from build123d import *

# Parameters (mm, degrees)
ESQUISSE1_R                                  = 5
BOSS_EXTRU_1_DEPTH                           = 5
CHAMBRAGE_POUR_VIS_T_TE_RONDE_BOMB_E_A_COUNT = 2
CHAMBRAGE_POUR_VIS_T_TE_RONDE_BOMB_E_A_PITCH = 152
CHAMBRAGE_POUR_VIS_T_TE_RONDE_BOMB_2_COUNT   = 2
CHAMBRAGE_POUR_VIS_T_TE_RONDE_BOMB_2_PITCH   = 111
CHAMBRAGE_POUR_VIS_T_TE_RONDE_BOMB_3_COUNT   = 2
CHAMBRAGE_POUR_VIS_T_TE_RONDE_BOMB_3_PITCH   = 188.215302247
CHAMBRAGE_POUR_VIS_T_TE_RONDE_BOMB_4_A_COUNT = 2
CHAMBRAGE_POUR_VIS_T_TE_RONDE_BOMB_4_A_PITCH = 152
CHAMBRAGE_POUR_VIS_T_TE_RONDE_BOMB_5_COUNT   = 2
CHAMBRAGE_POUR_VIS_T_TE_RONDE_BOMB_5_PITCH   = 111
CHAMBRAGE_POUR_VIS_T_TE_RONDE_BOMB_6_COUNT   = 2
CHAMBRAGE_POUR_VIS_T_TE_RONDE_BOMB_6_PITCH   = 188.215302247


with BuildPart() as part:
    # Esquisse1 → Boss.-Extru.1 (new body)
    with BuildSketch(Plane(origin=(0, 0, 0), x_dir=(1, 0, 0), z_dir=(0, 1, 0))):
        with Locations(Location((0, 0, 0), (0, 0, 270))):
            Circle(ESQUISSE1_R)
    extrude(amount=BOSS_EXTRU_1_DEPTH)

    # Esquisse3 → Chambrage pour vis _ t_te ronde bomb_e (revolve, cut)
    with BuildSketch(Plane(origin=(0, 11, -152), x_dir=(0, 0, 1), z_dir=(1, 0, 0))):
        Polygon((0, 0), (0, 6.839402285), (1.397, 6), (1.397, 1.8034), (2.77876, 1.8034), (2.77876, 0.635), (3.41376, 0), align=None)
    chambrage_pour_vis_t_te_ronde_bomb_e = revolve(axis=Axis((0, 17.35, -152), (0, -1, 0)), mode=Mode.SUBTRACT)

    # Chambrage pour vis _ t_te ronde bomb_e a: Chambrage pour vis _ t_te ronde bomb_e ×2
    with Locations(*[(0, 0, i * CHAMBRAGE_POUR_VIS_T_TE_RONDE_BOMB_E_A_PITCH) for i in range(1, CHAMBRAGE_POUR_VIS_T_TE_RONDE_BOMB_E_A_COUNT)]):
        add(chambrage_pour_vis_t_te_ronde_bomb_e, mode=Mode.SUBTRACT)

    # Chambrage pour vis _ t_te ronde bomb 2: Chambrage pour vis _ t_te ronde bomb_e ×2
    with Locations(*[(i * CHAMBRAGE_POUR_VIS_T_TE_RONDE_BOMB_2_PITCH, 0, 0) for i in range(1, CHAMBRAGE_POUR_VIS_T_TE_RONDE_BOMB_2_COUNT)]):
        add(chambrage_pour_vis_t_te_ronde_bomb_e, mode=Mode.SUBTRACT)

    # Chambrage pour vis _ t_te ronde bomb 3: Chambrage pour vis _ t_te ronde bomb_e ×2
    with Locations(*[Vector(0.5897501354816591, 0, 0.8075857711100195) * (i * CHAMBRAGE_POUR_VIS_T_TE_RONDE_BOMB_3_PITCH) for i in range(1, CHAMBRAGE_POUR_VIS_T_TE_RONDE_BOMB_3_COUNT)]):
        add(chambrage_pour_vis_t_te_ronde_bomb_e, mode=Mode.SUBTRACT)

    # Esquisse5 → Chambrage pour vis _ t_te ronde bomb 4 (revolve, cut)
    with BuildSketch(Plane(origin=(0, 11, 0), x_dir=(0, 0, 1), z_dir=(1, 0, 0))):
        Polygon((0, 0), (0, 6.839402285), (1.397, 6), (1.397, 1.8034), (2.77876, 1.8034), (2.77876, 0.635), (3.41376, 0), align=None)
    chambrage_pour_vis_t_te_ronde_bomb_4 = revolve(axis=Axis((0, 17.35, 0), (0, -1, 0)), mode=Mode.SUBTRACT)

    # Chambrage pour vis _ t_te ronde bomb 4 a: Chambrage pour vis _ t_te ronde bomb 4 ×2
    with Locations(*[Vector(-0.4987370820513642, 0, -0.8667533230319286) * (i * CHAMBRAGE_POUR_VIS_T_TE_RONDE_BOMB_4_A_PITCH) for i in range(1, CHAMBRAGE_POUR_VIS_T_TE_RONDE_BOMB_4_A_COUNT)]):
        add(chambrage_pour_vis_t_te_ronde_bomb_4, mode=Mode.SUBTRACT)

    # Chambrage pour vis _ t_te ronde bomb 5: Chambrage pour vis _ t_te ronde bomb 4 ×2
    with Locations(*[Vector(-0.8667533230319285, 0, 0.4987370820513645) * (i * CHAMBRAGE_POUR_VIS_T_TE_RONDE_BOMB_5_PITCH) for i in range(1, CHAMBRAGE_POUR_VIS_T_TE_RONDE_BOMB_5_COUNT)]):
        add(chambrage_pour_vis_t_te_ronde_bomb_4, mode=Mode.SUBTRACT)

    # Chambrage pour vis _ t_te ronde bomb 6: Chambrage pour vis _ t_te ronde bomb 4 ×2
    with Locations(*[Vector(-0.9139408606768702, 0, -0.40584738903339235) * (i * CHAMBRAGE_POUR_VIS_T_TE_RONDE_BOMB_6_PITCH) for i in range(1, CHAMBRAGE_POUR_VIS_T_TE_RONDE_BOMB_6_COUNT)]):
        add(chambrage_pour_vis_t_te_ronde_bomb_4, mode=Mode.SUBTRACT)


solid = part.part
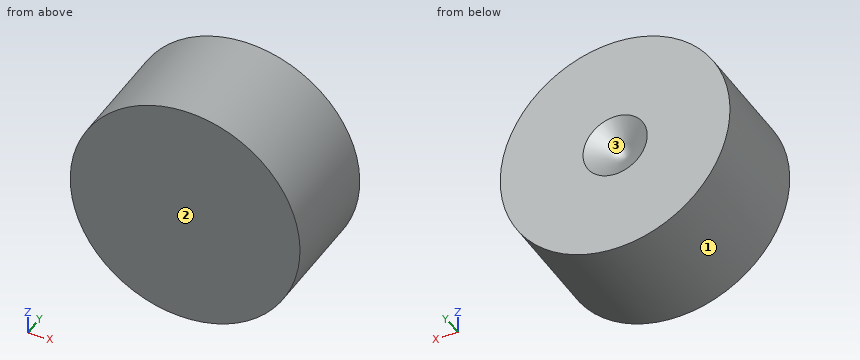
Model file for the job. Use its own axes, mm. Face numbers are marked on the shaded views. Give positions to 0.01 mm unless a question says otherwise; leave off trailing zeros. Order: outer loops, then holes, each group sorted by start corner. A loop starts at its lowest first (then second) coordinate and runs counter-clockwise, first axis right, second up. Notation, with made-up numbers: (46.5, 45) -> (65.5, 45) arc R22 ccw to (65.5, 65) -> close; hole circle Ø1 at (62, 77). An arc over 180 degrees is marked (long way). Use CSV: the item, a comma, the result in double quotes.
1. Band-saw the part on A-A, the plane y = 0.55. Give the cut face in (x, z), then the cut area to 3 significant figures.
Outcome:
outline,"circle Ø10 at (0, 0)"
area,"78.5 mm²"
2. Drop a flat-ended pin along its axis: pin 1 (1.5 mm diameter, centred on x = -3.5, y = 2.5, fed in from -Z). Give the stop position or say it passes through.
Outcome:
pin 1,"z = -4.18"
3. Band-saw the part on C-C, the plane z = 2.25. Give the cut face in (x, y), then the cut area to 3 significant figures.
Outcome:
outline,"(-4.47, 0) -> (4.47, 0) -> (4.47, 5) -> (-4.47, 5) -> close"
area,"44.7 mm²"
4. Band-saw the part on B-B, the plane x = 2.75. Give the cut face in (y, z).
Outcome:
outline,"(0, -4.18) -> (5, -4.18) -> (5, 4.18) -> (0, 4.18) -> close"
5. Mould opens along X. For the marked faces 1, 2 and 3 say: +X half, -X half, draft (parallel to the pull), parting line (faces both ways), or undercut.
Outcome:
face 1,"parting line"
face 2,"draft"
face 3,"undercut"
6. Drill centre lines: line 1 along Z through (x, y) = (4, 2.05); line 2 along X through (y, z) = (2.45, 2.75); line 3 along X through (y, z) = (1.85, 1). Where is each one in solid material? Low to high. Write a range as from..to.
Outcome:
line 1,"-3..3"
line 2,"-4.18..4.18"
line 3,"-4.9..4.9"
